Model file for the job. Use its own axes, mm. A direction names the side the tool comes from. Coordinates: 2 decimals unless noted, no trailing zeros. Write each loop counter-clockwise with the first axis right and the second up, starting at its lowest first coordinate (ties: lowest second). Pieces come first, ordered by that corner, then holes.
Q1. Band-saw the part on B-B, the plane x = 0. Write the cut outline in (y, z) (1 decimal), plus the area to 3 significant figures.
Q2. Drill centre lines: probe 1 along Z at (x, y) = (0, 1.25) (3 decimals); probe 2 along X at (y, z) = (2.3, -5); probe 3 along Z at (x, y) = (-1, 1.6). Where is each one in solid material? Low to high.
Q3. Band-saw the part on D-D, the plane z = -34.5. Write the cut outline in (x, y), plus the area to 3 significant figures.
Q4. Band-saw the part on A-A, the plane z = -50. Write the cut outline in (x, y) (1 decimal), plus the area to 3 significant figures.
Q5. Band-saw the part on C-C, the plane x = 4. Write the cut outline in (y, z).
Q6. Which spindle directions (+Z, -Z, +X, -X, +Y, -Y) get a long thin tool onto all of the face, cutting with end or side? Do faces 4 (the flat face through (7.5, 2, -15)), 5 (the flat face through (0, 2, 0)), 6 (the flat face through (-7.5, 2, -15)). Say none if no direction does.
Q7. Pull direction X, two halves, no side cores. Call faces 1 (the flat face through (0, 0, -33)), 2 (the cylindrical face through (0, 2, -65)), 3 (the cylindrical face through (-2.06, 2.35, -40.7)): released by +X, released by -X, zero draft, split by the parting line, or undercut.
Q8. Pin check, flat tips, straight feed: P1, Ø1.5, axis at x = 10.5, y = 3.5, coming from the -Z side; P2, Ø2.5, axis at y = 3, z = -9, coming from the +X side; P3, Ø2, axis at y = 4, z = -31, coming from the -X side. Stop position of each tip, or through.
from build123d import *

# Parameters (mm, degrees)
SKETCH1_R           = 9.525
SKETCH1_R_2         = 1.6
BOSS_EXTRUDE2_DEPTH = 4.7625


with BuildPart() as part:
    # Sketch1 → Boss-Extrude2 (new body)
    with BuildSketch(Plane(origin=(0, 0, 0), x_dir=(1, 0, 0), z_dir=(0, 1, 0))):
        with BuildLine():
            Line((-7.5, 0), (7.5, 0))
            Line((7.5, 0), (7.5, 30))
            ThreePointArc((7.5, 30), (8.481591846, 35.413153058), (11.301369863, 40.136986301))
            ThreePointArc((11.301369863, 40.136986301), (0, 65), (-11.301369863, 40.136986301))
            ThreePointArc((-11.301369863, 40.136986301), (-8.481591846, 35.413153058), (-7.5, 30))
            Line((-7.5, 30), (-7.5, 0))
        make_face()
        with Locations((0, 50)):
            Circle(SKETCH1_R, mode=Mode.SUBTRACT)
        with Locations((0, 5)):
            Circle(SKETCH1_R_2, mode=Mode.SUBTRACT)
        with Locations((0, 25)):
            Circle(SKETCH1_R_2, mode=Mode.SUBTRACT)
    extrude(amount=BOSS_EXTRUDE2_DEPTH)


solid = part.part
Answer sheet:
1. outline: (0, -65) - (4.8, -65) - (4.8, -59.5) - (0, -59.5) - close; (0, -40.5) - (4.8, -40.5) - (4.8, -26.6) - (0, -26.6) - close; (0, -23.4) - (4.8, -23.4) - (4.8, -6.6) - (0, -6.6) - close; (0, -3.4) - (4.8, -3.4) - (4.8, 0) - (0, 0) - close
1. area: 188 mm2
2. probe 1: z = -65 to -59.525, -40.475 to -26.6, -23.4 to -6.6, -3.4 to 0
2. probe 2: x = -7.5 to -1.6, 1.6 to 7.5
2. probe 3: z = -64.97 to -59.47, -40.53 to -26.25, -23.75 to -6.25, -3.75 to 0
3. outline: (-8.17, 0) - (8.17, 0) - (8.17, 4.76) - (-8.17, 4.76) - close
3. area: 77.8 mm2
4. outline: (-15, 0) - (-9.5, 0) - (-9.5, 4.8) - (-15, 4.8) - close; (9.5, 0) - (15, 0) - (15, 4.8) - (9.5, 4.8) - close
4. area: 52.1 mm2
5. outline: (0, -64.46) - (4.76, -64.46) - (4.76, -58.64) - (0, -58.64) - close; (0, -41.36) - (4.76, -41.36) - (4.76, 0) - (0, 0) - close
6. face 4: +Z, +X, +Y, -Y
6. face 5: +Z, +X, -X, +Y, -Y
6. face 6: +Z, -X, +Y, -Y
7. face 1: zero draft
7. face 2: split by the parting line
7. face 3: undercut
8. P1: stops at z = -61.4
8. P2: stops at x = 7.5
8. P3: stops at x = -7.63
